from build123d import *

# Parameters (mm, degrees)
F0_R     = 3.45
F0_R_2   = 2.35
F1_DEPTH = 18
F2_R     = 8
F2_R_2   = 3.45
F3_DEPTH = 10
F4_R     = 1
F5_R     = 1


with BuildPart() as f1:
    # F0 (on Top) → F1 (new body)
    with BuildSketch(Plane.XY):
        Circle(F0_R)
        Circle(F0_R_2, mode=Mode.SUBTRACT)
    extrude(amount=F1_DEPTH)

    # F2 (on Top) → F3 (join)
    with BuildSketch(Plane.XY):
        Circle(F2_R)
        Circle(F2_R_2, mode=Mode.SUBTRACT)
    extrude(amount=F3_DEPTH)

    # F4
    f4_edges = [f1.edges().sort_by_distance(p)[0] for p in [
        (-3.45, 0, 18),
    ]]
    fillet(f4_edges, radius=F4_R)

    # F5
    f5_edges = [f1.edges().sort_by_distance(p)[0] for p in [
        (-2.35, 0, 0),
    ]]
    fillet(f5_edges, radius=F5_R)


solid = f1.part
Read the model definition and answer for the solid it produces. Units are mm, in the model's axes. A direction names the side the tool comes from. Round coordinates to 2 decimals unless told otherwise and drop trailing zeros. Write each loop counter-clockwise with the first axis right and the second up, starting at its lowest first coordinate (ties: lowest second). Pieces come first, ordered by that corner, then holes. Notation, with made-up numbers: M 64,62 L 71,62 A17 ccw 71,94 Z; hole C 75,16 d5. An arc over 180 degrees is marked long. Use a Markdown table: item, result.
1) Straight lines are drawn through the part: line 1 along Y through (x, z) = (0, 9.5); line 2 along Y through (x, z) = (0, 13.5); line 3 along Z through (x, y) = (-1, -5.5). For each, find the intervals that lie inside material, in ascending order. Write a range as [from, to].
Answers follow:
| item | result |
|---|---|
| line 1 | y = [-8, -2.35], [2.35, 8] |
| line 2 | y = [-3.45, -2.35], [2.35, 3.45] |
| line 3 | z = [0, 10] |
2) A tool of negligible diameter and unlimited length cuts with its end or side. For faces 1 (the cylindrical face through (-1.73, -7.81, 4.93)), 2 (the flat face through (3, -2, 10)), from which of +Z, -Z, +X, -X, +Y, -Y can it reach the whole face along a straight path? Write none if from no direction.
Answers follow:
| item | result |
|---|---|
| face 1 | +Z, -Z |
| face 2 | +Z |
3) The part is cut by section D-D (z = 6.5). Write down the section's boundary in (x, y).
Answers follow:
| item | result |
|---|---|
| outline | C 0,0 d16; hole C 0,0 d4.7 |
4) The part is cut by section C-C (z = 16). Write down the section's boundary in (x, y).
Answers follow:
| item | result |
|---|---|
| outline | C 0,0 d6.9; hole C 0,0 d4.7 |
5) The part is cut by section A-A (y = 0). Write down the section's boundary in (x, z), plus the area to 3 significant figures.
Answers follow:
| item | result |
|---|---|
| outline | M -8,0 L -3.35,0 A1 ccw -2.35,1 L -2.35,18 L -2.45,18 A1 ccw -3.45,17 L -3.45,10 L -8,10 Z; M 2.35,1 A1 ccw 3.35,0 L 8,0 L 8,10 L 3.45,10 L 3.45,17 A1 ccw 2.45,18 L 2.35,18 Z |
| area | 130 mm2 |
6) Flat-ended cylindrical pins translate along their axes: pin 1 (1.5 mm diameter, centred on x = -1.5, z = 4, fed in from +Y); pin 2 (6 mm diameter, centred on x = 6, z = 10.5, fed in from -Y); pin 3 (2 mm diameter, centred on y = 5, z = 2.5, fed in from +X). Find the tip coordinate at first contact, or state that the pin passes through.
Answers follow:
| item | result |
|---|---|
| pin 1 | stops at y = 7.96 |
| pin 2 | stops at y = -7.4 |
| pin 3 | stops at x = 6.93 |
7) For a pull along Y with two mould halves and no side action, classify faces 3 (the flat face through (3, -2, 0)), 4 (the cylindrical face through (-0.45, 3.42, 13.45)), 5 (the cylindrical face through (-0.509, -2.294, 9.381)) as pulls with the +Y half, pulls with the -Y half, needs draft (parallel to the pull), parting line crosses it, or undercut.
Answers follow:
| item | result |
|---|---|
| face 3 | needs draft |
| face 4 | parting line crosses it |
| face 5 | undercut |
